Geometry check sheet. Reference: the model listing, model coordinates, mm. A direction names the side the tool comes from. Round coordinates to 2 decimals unless told otherwise and drop trailing zeros. Order: outer loops, then holes, each group sorted by start corner. A loop starts at its lowest first (then second) coordinate and runs counter-clockwise, first axis right, second up.
(1) Sectioned sample at B-B (z = -4.5). Record the boundary of the cut face in (x, y).
(2) Sectioned sample at C-C (x = 4.75). Record the boundary of the cut face in (y, z), plus the area to 3 significant figures.
(3) Release check for a two-part mould opening along Z. For faces 1 (the face through (0, 163, -10)), 2 (the face through (10, 163, -18.55)), 3 (the face through (10, 163, -20)) record: +Z half, -Z half, draft (parallel to the pull), parting line (faces both ways), or undercut.
(4) Material ranges on line 1 along X through (y, z) = (278, -12); line 2 along Z through (x, y) = (10, 100); line 3 along X through (y, z) = (340, -19.55), recorded low to high.
(5) Sectioned sample at A-A (y = 229.5). Record the boundary of the cut face in (x, z).
(6) Set-up check for faces 4 (the face through (1.45, 163, -10)), 5 (the face through (10, 163, 0)): record each of +Z, -Z, +X, -X, +Y, -Y from which the full face is reachable in a straight line by a thin tool's end or side.
from build123d import *

# Parameters (mm, degrees)
SKETCH1_W           = 20
SKETCH1_H           = 20
SKETCH1_W_2         = 17.1
SKETCH1_H_2         = 17.1
BOSS_EXTRUDE1_DEPTH = 350
SKETCH2_R           = 2.05
CUT_EXTRUDE1_DEPTH  = 21
SKETCH3_R           = 2.05
CUT_EXTRUDE2_DEPTH  = 21
SKETCH4_W           = 20
SKETCH4_H           = 20
SKETCH4_W_2         = 17.1
SKETCH4_H_2         = 17.1
BOSS_EXTRUDE2_DEPTH = 30


with BuildPart() as part:
    # Sketch1 → Boss-Extrude1 (new body)
    with BuildSketch(Plane(origin=(0, 0, 0), x_dir=(1, 0, 0), z_dir=(0, 1, 0))):
        with Locations((10, 10)):
            Rectangle(SKETCH1_W, SKETCH1_H)
        with Locations((10, 10)):
            Rectangle(SKETCH1_W_2, SKETCH1_H_2, mode=Mode.SUBTRACT)
    extrude(amount=BOSS_EXTRUDE1_DEPTH)

    # Sketch2 → Cut-Extrude1 (cut, through all)
    with BuildSketch(Plane(origin=(0, 0, -20), x_dir=(-1, 0, 0), z_dir=(0, 0, -1))):
        with Locations((-10, 340)):
            Circle(SKETCH2_R)
        with Locations((-10, 310)):
            Circle(SKETCH2_R)
        with Locations((-10, 20)):
            Circle(SKETCH2_R)
        with Locations((-10, 5)):
            Circle(SKETCH2_R)
    extrude(amount=-CUT_EXTRUDE1_DEPTH, mode=Mode.SUBTRACT)

    # Sketch3 → Cut-Extrude2 (cut, through all)
    with BuildSketch(Plane(origin=(0, 0, -20), x_dir=(-1, 0, 0), z_dir=(0, 0, -1))):
        with Locations((-10, 103)):
            Circle(SKETCH3_R)
        with Locations((-10, 53)):
            Circle(SKETCH3_R)
    extrude(amount=-CUT_EXTRUDE2_DEPTH, mode=Mode.SUBTRACT)

    # Sketch4 → Boss-Extrude2 (add)
    with BuildSketch(Plane.XZ):
        with Locations((10, -10)):
            Rectangle(SKETCH4_W, SKETCH4_H)
        with Locations((10, -10)):
            Rectangle(SKETCH4_W_2, SKETCH4_H_2, mode=Mode.SUBTRACT)
    extrude(amount=BOSS_EXTRUDE2_DEPTH)


solid = part.part
Answer below:
1. outline: (0, -30) - (1.45, -30) - (1.45, 350) - (0, 350) - close; (18.55, -30) - (20, -30) - (20, 350) - (18.55, 350) - close
2. outline: (-30, -20) - (350, -20) - (350, -18.55) - (-30, -18.55) - close; (-30, -1.45) - (350, -1.45) - (350, 0) - (-30, 0) - close
2. area: 1,100 mm2
3. face 1: draft
3. face 2: undercut
3. face 3: -Z half
4. line 1: x = 0 to 1.45, 18.55 to 20
4. line 2: z = -20 to -18.55, -1.45 to 0
4. line 3: x = 0 to 7.95, 12.05 to 20
5. outline: (0, -20) - (20, -20) - (20, 0) - (0, 0) - close; hole (1.45, -18.55) - (18.55, -18.55) - (18.55, -1.45) - (1.45, -1.45) - close
6. face 4: +Y, -Y
6. face 5: +Z, +X, -X, +Y, -Y
